Can you work these out from the model? Positions are in its coordinate system, mm. Face numbers are marked on the shaded views. A direction names the side the tool comes from. Round coordinates to 2 decimals unless told otherwise and drop trailing zeros. Write each loop counter-clockwise with the first axis right and the second up, starting at its lowest first coordinate (ties: lowest second). Pieces come first, ordered by that corner, then holes. Notation, with made-up numbers: (13.25, 7) -> (42.25, 7) arc R8 cw to (42.25, 11) -> close; hole circle Ø8 at (77, 82). An arc over 180 degrees is marked (long way). Write item = value, one per line. Start each with the question number.
1) If I drill on line 1 (Y direction, x = 0, z = 4.75); line 2 (X direction, y = -30.5, z = 14); line 3 (Y direction, x = 44, z = 18), over which ranges is the centre line in solid material (lowest first)?
2) I'm going to push flat-ended pins straight in: pin 1 (18 mm diameter, centred on x = 0, y = 0, fed in from -Z); pin 2 (2 mm diameter, centred on y = -22, z = 14, fed in from -X); pin 3 (13 mm diameter, centred on x = 20, y = 50, fed in from +Z); pin 4 (5 mm diameter, centred on x = -43, z = 13, fed in from +Y). Where does each tip first touch, or does it pass through?
3) Imagine slicing it at C-C, the plane x = 33. Please give me the cut outline in (y, z).
4) Thinking about a two-plate mould opening in X: for the marked faces 4, 5 and 6, which applies, +X half, -X half, draft (parallel to the pull), parting line (faces both ways), or undercut?
5) For the marked faces 1, 2 and 3, which set-ups out of +Z, -Z, +X, -X, +Y, -Y let a thin tool reach every point of the face, with its end or its side?
6) Imagine slicing it at A-A, the plane y = 56.5. Please give me the cut outline in (x, z).
7) Imagine slicing it at B-B, the plane z = 12.75. Please give me the cut outline in (x, y).
from build123d import *

# Parameters (mm, degrees)
SKETCH1_R           = 5
BOSS_EXTRUDE1_DEPTH = 10
BOSS_EXTRUDE2_DEPTH = 20


with BuildPart() as part:
    # Sketch1 → Boss-Extrude1 (new body)
    with BuildSketch(Plane.XY):
        with BuildLine():
            ThreePointArc((-15.811936897, -34.554054054), (0, -21), (15.811936897, -34.554054054))
            ThreePointArc((15.811936897, -34.554054054), (31.975409318, -20.532247781), (38, 0))
            Line((38, 0), (48, 0))
            Line((48, 0), (28.501872629, 59.361797724))
            ThreePointArc((28.501872629, 59.361797724), (0, 80), (-28.501872629, 59.361797724))
            Line((-28.501872629, 59.361797724), (-48, 0))
            Line((-48, 0), (-38, 0))
            ThreePointArc((-38, 0), (-31.975409318, -20.532247781), (-15.811936897, -34.554054054))
        make_face()
        with Locations((20, 50)):
            Circle(SKETCH1_R, mode=Mode.SUBTRACT)
        with Locations((14.142135624, 64.142135624)):
            Circle(SKETCH1_R, mode=Mode.SUBTRACT)
        with Locations((0, 70)):
            Circle(SKETCH1_R, mode=Mode.SUBTRACT)
        with Locations((-14.142135624, 64.142135624)):
            Circle(SKETCH1_R, mode=Mode.SUBTRACT)
        with Locations((-20, 50)):
            Circle(SKETCH1_R, mode=Mode.SUBTRACT)
        with BuildLine():
            ThreePointArc((7.921212028, 51.12), (0, 58), (-7.921212028, 51.12))
            Line((-7.921212028, 51.12), (-14.852272553, 2.1))
            ThreePointArc((-14.852272553, 2.1), (0, -15), (14.852272553, 2.1))
            Line((14.852272553, 2.1), (7.921212028, 51.12))
        make_face(mode=Mode.SUBTRACT)
    extrude(amount=BOSS_EXTRUDE1_DEPTH)

    # Sketch1_3 → Boss-Extrude2 (add)
    with BuildSketch(Plane.XY):
        with BuildLine():
            ThreePointArc((15.811936897, -34.554054054), (31.975409318, -20.532247781), (38, 0))
            Line((38, 0), (48, 0))
            ThreePointArc((48, 0), (0, -48), (-48, 0))
            Line((-48, 0), (-38, 0))
            ThreePointArc((-38, 0), (-31.975409318, -20.532247781), (-15.811936897, -34.554054054))
            ThreePointArc((-15.811936897, -34.554054054), (0, -21), (15.811936897, -34.554054054))
        make_face()
    extrude(amount=BOSS_EXTRUDE2_DEPTH)


solid = part.part
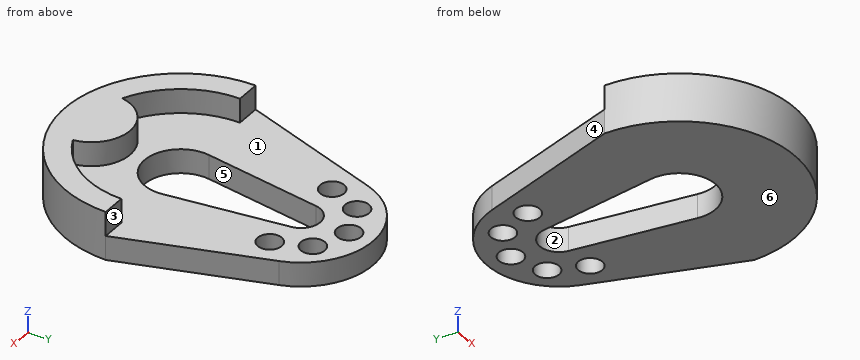
Reported:
q1.line_1 = -48 to -15, 58 to 65, 75 to 80
q1.line_2 = -37.06 to -22.67, -14.62 to 14.62, 22.67 to 37.06
q1.line_3 = -19.18 to 0
q2.pin_1 = through
q2.pin_2 = -43.16
q2.pin_3 = 10
q2.pin_4 = 0
q3.outline = (-34.86, 0) -> (45.67, 0) -> (45.67, 10) -> (-18.84, 10) -> (-18.84, 20) -> (-34.86, 20) -> close
q4.face_4 = -X half
q4.face_5 = undercut
q4.face_6 = draft
q5.face_1 = +Z, +Y
q5.face_2 = +Z, -Z
q5.face_3 = +Z, +X, -X, +Y
q6.outline = (-29.44, 0) -> (-4.66, 0) -> (-4.66, 10) -> (-29.44, 10) -> close; (4.66, 0) -> (29.44, 0) -> (29.44, 10) -> (4.66, 10) -> close
q7.outline = (-48, 0) arc R48 ccw to (48, 0) -> (38, 0) arc R38 cw to (15.81, -34.55) arc R16 ccw to (-15.81, -34.55) arc R38 cw to (-38, 0) -> close
